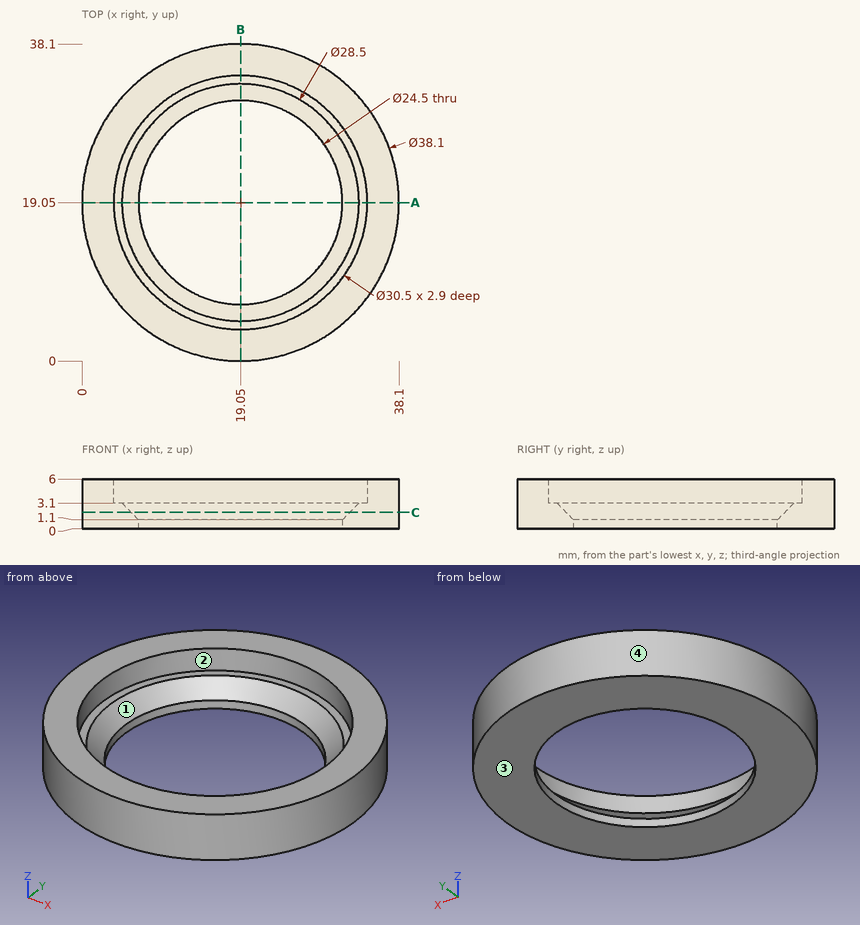
The drawing under review shows one solid part. Ordinate dimensions are in mm from its lowest x, y, z. Round coordinates to 2 decimals unless told otherwise and drop trailing zeros. Loops run counter-clockwise (first coordinate to the right, second up) from the corner with the lowest first, then second, coordinate; pieces in that order, holes last. Notation, with made-up numbers: (28.5, -1.5) - (36.5, -1.5) arc R23 cw to (36.5, 25.5) - close; hole circle Ø1 at (21, 68). An arc over 180 degrees is marked (long way). Put each result on its own line as item: value. Start each with the question number.
1. Consider section A-A on y = 19.05. State the section outline as (x, z) points, plus the area to 3 significant figures.
2. Mouldability with a two-part tool opening along Y and no side actions: class the marked faces 1, 2, 3 and 4 as +Y half, -Y half, draft (parallel to the pull), parting line (faces both ways), or undercut.
3. For probe 1 along Y at (x, z) = (19.05, 0.4); probe 2 along Y at (x, z) = (19.05, 5.2); probe 3 along X at (y, z) = (10.5, 1.05), list the stretches that pass through material, from the lowest coordinate up. Write a range as [from, to].
4. Insertion check: P1, Ø5, axis at x = 12.5, y = 9.5, coming from the +Z side; P2, Ø3, axis at x = 9, z = 5, coming from the -Y side; P3, Ø8, axis at x = 32.5, y = 30, coming from the -Z side; P4, Ø1.5, axis at x = 24, z = 2, coming from the +Y side. Each pin has a flat end and moves straight along its axis. Give the tip position at first contact, or say it passes through.
5. Consider section C-C on z = 2. State the section outline as (x, y) points, plus the area to 3 significant figures.
Result sheet:
1. outline: (0, 0) - (6.8, 0) - (6.8, 1.1) - (4.8, 3.1) - (3.8, 3.1) - (3.8, 6) - (0, 6) - close; (31.3, 0) - (38.1, 0) - (38.1, 6) - (34.3, 6) - (34.3, 3.1) - (33.3, 3.1) - (31.3, 1.1) - close
1. area: 60.2 mm^2
2. face 1: undercut
2. face 2: undercut
2. face 3: draft
2. face 4: parting line
3. probe 1: [0, 6.8], [31.3, 38.1]
3. probe 2: [0, 3.8], [34.3, 38.1]
3. probe 3: [2.03, 10.28], [27.82, 36.07]
4. P1: z = 2.93
4. P2: y = 2.03
4. P3: z = 0
4. P4: y = 37.63
5. outline: circle Ø38.1 at (19.05, 19.05); hole circle Ø26.3 at (19.05, 19.05)
5. area: 597 mm^2
